from build123d import *

# Parameters (mm, degrees)
F0_W     = 100
F0_H     = 100
F0_W_2   = 96
F0_H_2   = 96
F1_DEPTH = 75
F0_R     = 11.5
F2_DEPTH = 2
F4_DEPTH = 10
F5_R     = 2
F6_DEPTH = 10


with BuildPart() as f1:
    # F0 (on Top) → F1 (new body)
    with BuildSketch(Plane.XY):
        Rectangle(F0_W, F0_H)
        Rectangle(F0_W_2, F0_H_2, mode=Mode.SUBTRACT)
    extrude(amount=F1_DEPTH)

    # F0 (on Top) → F2 (join)
    with BuildSketch(Plane.XY):
        Rectangle(F0_W_2, F0_H_2)
        with Locations((28, 28)):
            Circle(F0_R, mode=Mode.SUBTRACT)
    extrude(amount=F2_DEPTH)

    # F3 (on face) → F4 (join)
    with BuildSketch(Plane.XY.offset(75)):
        with BuildLine():
            Line((46.5, 48), (40.5, 48))
            ThreePointArc((40.5, 48), (42.696699, 42.696699), (48, 40.5))
            Line((48, 40.5), (48, 46.5))
            ThreePointArc((48, 46.5), (45.43934, 45.43934), (46.5, 48))
        make_face()
        with BuildLine():
            Line((48, -46.5), (48, -40.5))
            ThreePointArc((48, -40.5), (42.696699, -42.696699), (40.5, -48))
            Line((40.5, -48), (46.5, -48))
            ThreePointArc((46.5, -48), (45.43934, -45.43934), (48, -46.5))
        make_face()
        with BuildLine():
            ThreePointArc((-40.5, -48), (-42.696699, -42.696699), (-48, -40.5))
            Line((-48, -40.5), (-48, -46.5))
            ThreePointArc((-48, -46.5), (-46.5, -45), (-45, -46.5))
            ThreePointArc((-45, -46.5), (-45.43934, -47.56066), (-46.5, -48))
            Line((-46.5, -48), (-40.5, -48))
        make_face()
        with BuildLine():
            ThreePointArc((-48, 40.5), (-42.696699, 42.696699), (-40.5, 48))
            Line((-40.5, 48), (-46.5, 48))
            ThreePointArc((-46.5, 48), (-45.43934, 47.56066), (-45, 46.5))
            ThreePointArc((-45, 46.5), (-46.5, 45), (-48, 46.5))
            Line((-48, 46.5), (-48, 40.5))
        make_face()
    extrude(amount=-F4_DEPTH)

    # F5
    f5_edges = [f1.edges().sort_by_distance(p)[0] for p in [
        (-42.696699, -42.696699, 65),
        (-42.696699, 42.696699, 65),
        (42.696699, 42.696699, 65),
        (42.696699, -42.696699, 65),
    ]]
    fillet(f5_edges, radius=F5_R)

    # F3 (on face) → F6 (cut)
    with BuildSketch(Plane.XY.offset(75)):
        with BuildLine():
            ThreePointArc((-45, 46.5), (-45.43934, 47.56066), (-46.5, 48))
            ThreePointArc((-46.5, 48), (-47.56066, 47.56066), (-48, 46.5))
            ThreePointArc((-48, 46.5), (-46.5, 45), (-45, 46.5))
        make_face()
        with BuildLine():
            ThreePointArc((48, 46.5), (47.56066, 47.56066), (46.5, 48))
            ThreePointArc((46.5, 48), (45.43934, 45.43934), (48, 46.5))
        make_face()
        with BuildLine():
            ThreePointArc((46.5, -48), (47.56066, -47.56066), (48, -46.5))
            ThreePointArc((48, -46.5), (45.43934, -45.43934), (46.5, -48))
        make_face()
        with BuildLine():
            ThreePointArc((-45, -46.5), (-46.5, -45), (-48, -46.5))
            ThreePointArc((-48, -46.5), (-47.56066, -47.56066), (-46.5, -48))
            ThreePointArc((-46.5, -48), (-45.43934, -47.56066), (-45, -46.5))
        make_face()
    extrude(amount=-F6_DEPTH, mode=Mode.SUBTRACT)


solid = f1.part
Geometry check sheet. Reference: the model listing, model coordinates, mm. A direction names the side the tool comes from. Round coordinates to 2 decimals unless told otherwise and drop trailing zeros. Order: outer loops, then holes, each group sorted by start corner. A loop starts at its lowest first (then second) coordinate and runs counter-clockwise, first axis right, second up. Notation, with made-up numbers: (-3.75, 32) - (10.25, 32) arc R34 cw to (10.25, 71) - close; hole circle Ø6 at (34, 9). An arc over 180 degrees is marked (long way). One line per question, with ' | ' between items. Start each with the question number.
(1) Sectioned sample at A-A on y = 28. Record the cut outline in (x, z), and give its area (3 significant figures).
(2) Thickness scan on L1, parallel to Y at x = 38, z = 13.5; L2, parallel to X at y = 46.5, z = 68.5. Record the ranges inside material, lowest first. Write a range as [from, to].
(3) Release check for a two-part mould opening along X. For faces 4 (the flat face through (-50, -1, 37)), 5 (the flat face through (50, -1, 37)), 6 (the flat face through (-48, -1, 38)) record: released by +X, released by -X, zero draft, split by the parting line, or undercut.
(4) Sectioned sample at C-C on z = 25.5. Record the cut outline in (x, y).
(5) Sectioned sample at B-B on x = -14. Record the cut outline in (y, z), and give its area (3 significant figures).
(6) Access from +Z, -Z, +X, -X, +Y, -Y to the whole of each face (thin tool, end or side, straight path). Record for faces 1 (the cylindrical face through (18.874, 21.002, 0.986)), 2 (the cylindrical face through (-42.755, 42.639, 71.056)), 3 (the flat face through (-45, 45, 65)).
(7) Depth check by flat-ended pin: pin 1 Ø6 at (x, y) = (-21.5, 4.5) entering from -Z; pin 2 Ø2.5 at (x, y) = (46.5, -46.5) entering from +Z. Enter the tip coordinate at first touch or a pass-through.
Conclusion:
1) outline: (-50, 0) - (16.5, 0) - (16.5, 2) - (-48, 2) - (-48, 75) - (-50, 75) - close; (39.5, 0) - (50, 0) - (50, 75) - (48, 75) - (48, 2) - (39.5, 2) - close | area: 446 mm2
2) L1: y = [-50, -48], [48, 50] | L2: x = [-50, -48], [-45, -40.65], [40.65, 45], [48, 50]
3) face 4: released by -X | face 5: released by +X | face 6: undercut
4) outline: (-50, -50) - (50, -50) - (50, 50) - (-50, 50) - close; hole (-48, -48) - (48, -48) - (48, 48) - (-48, 48) - close
5) outline: (-50, 0) - (50, 0) - (50, 75) - (48, 75) - (48, 2) - (-48, 2) - (-48, 75) - (-50, 75) - close | area: 492 mm2
6) face 1: +Z, -Z | face 2: +Z | face 3: none
7) pin 1: stops at z = 0 | pin 2: stops at z = 2
